Autodesk Inventor part; units mm, degrees
ref_plane "YZ Plane" through (0, 0, 0) normal (1, 0, 0) x (0, 1, 0)
ref_plane "XZ Plane" through (0, 0, 0) normal (0, 1, 0) x (-1, 0, 0)
ref_plane "XY Plane" through (0, 0, 0) normal (0, 0, 1) x (1, 0, 0)
sketch "Sketch1" plane through (0, 0, 0) normal (0, 1, 0) x (-1, 0, 0)
  circle A0 centre (0, 0) radius 30
  dimension "Stand_Diameter" = 60
extrude "Extrusion1" add sketch "Sketch1" along normal blind 70
sketch "Sketch2" plane through (0, 70, 0) normal (0, 1, 0) x (1, 0, 0)
  circle A0 centre (0, 0) radius 30
  circle A1 centre (0, 0) radius 17.5
  dimension "d5" = 35
extrude "Extrusion2" cut sketch "Sketch2" against normal blind 8 contours A1
chamfer "Chamfer1" distance 2 angle 45 2 edges at (30, 70, 0) (30, 0, 0)
properties part number "StandGreen" material "Wood (Oak)"
Check sheet for the modelled part. Datum: model origin and axes. Units: mm. A direction names the side the tool comes from. Round coordinates to 2 decimals unless told otherwise and drop trailing zeros. Loops run counter-clockwise (first coordinate to the right, second up) from the corner with the lowest first, then second, coordinate; pieces in that order, holes last. Notation, with made-up numbers: (83, 62.25) -> (117, 62.25) arc R24 ccw to (117, 76.25) -> close; hole circle Ø2 at (56, 5). An arc over 180 degrees is marked (long way). Put each result on its own line as item: value. Start each with the question number.
1. Scan lines: probe 1 along Z at (x, y) = (0, 66); probe 2 along Y at (x, z) = (-12, 4.5); probe 3 along X at (y, z) = (23.5, -1). Record each from-to range of solid material in increasing order.
2. Section check A-A (z = 0). Enter the section's corners in (x, y).
3. Access from +Z, -Z, +X, -X, +Y, -Y to the whole of each face (thin tool, end or side, straight path). Record for faces 4 (the face through (-13.887, 66.056, 10.648)), 5 (the face through (29.97, 34.54, -1.32)).
4. Section check C-C (y = 64.5). Enter the section's corners in (x, z), plus the area to 3 significant figures.
5. Section check D-D (y = 49.5). Enter the section's corners in (x, z).
6. Section check B-B (x = 0). Enter the section's corners in (y, z), plus the area to 3 significant figures.
7. Draft check along X on faces 1 (the face through (6.1, 0.13, -27.46)), 2 (the face through (0, 62, 0)), 3 (the face through (0, 0, 0)). Enter one of: +X half, -X half, draft (parallel to the pull), parting line (faces both ways), or undercut.
8. Gauge pin test, flat ends, axial feed: pin 1 (6 mm diameter, centred on y = 48, z = 16, fed in from +X); pin 2 (4 mm diameter, centred on y = 62, z = -23.5, fed in from -X); pin 3 (1.5 mm diameter, centred on x = -11.5, z = -11.5, fed in from +Y). Record the tip position at first contact, or that the pin passes through.
Findings:
1. probe 1: z = -30 to -17.5, 17.5 to 30
1. probe 2: y = 0 to 62
1. probe 3: x = -29.98 to 29.98
2. outline: (-30, 2) -> (-28, 0) -> (28, 0) -> (30, 2) -> (30, 68) -> (28, 70) -> (17.5, 70) -> (17.5, 62) -> (-17.5, 62) -> (-17.5, 70) -> (-28, 70) -> (-30, 68) -> close
3. face 4: +Y
3. face 5: +Y, -Y
4. outline: circle Ø60 at (0, 0); hole circle Ø35 at (0, 0)
4. area: 1,870 mm^2
5. outline: circle Ø60 at (0, 0)
6. outline: (0, -28) -> (2, -30) -> (68, -30) -> (70, -28) -> (70, -17.5) -> (62, -17.5) -> (62, 17.5) -> (70, 17.5) -> (70, 28) -> (68, 30) -> (2, 30) -> (0, 28) -> close
6. area: 3,910 mm^2
7. face 1: parting line
7. face 2: undercut
7. face 3: draft
8. pin 1: stops at x = 27.04
8. pin 2: stops at x = -20.92
8. pin 3: stops at y = 62
